Part model, mm, in its own coordinate system. Face numbers are marked on the shaded views. A direction names the side the tool comes from. Round coordinates to 2 decimals unless told otherwise and drop trailing zeros. Write each loop counter-clockwise with the first axis right and the second up, starting at its lowest first coordinate (ties: lowest second). Pieces come first, ordered by that corner, then holes.
1) Flat gauge pins, fed straight in: pin 1 (2.5 mm diameter, centred on x = -23.5, y = 23.5, fed in from -Z); pin 2 (10 mm diameter, centred on y = 4, z = 13.5, fed in from +X) (3 decimals); pin 3 (1.5 mm diameter, centred on x = -2.5, z = -27.5, fed in from +Y); pin 4 (8 mm diameter, centred on y = 6.5, z = -10.5, fed in from -X). Where does each tip first touch, or does it go through?
2) Which spindle directions (+Z, -Z, +X, -X, +Y, -Y) get a long thin tool onto all of the face, cutting with end or side? Do the marked faces 5, 6, 7 and 8. Say none if no direction does.
3) Saw through at B-B on x = 15.5. Write the cut outline in (y, z).
4) Pull direction Z, two halves, no side cores. Call the marked faces 1, 2, 3 and 4: +Z half, -Z half, draft (parallel to the pull), parting line (faces both ways), or undercut.
5) Saw through at D-D on z = 13.5. Write the cut outline in (x, y) (3 decimals), and give its area (3 significant figures).
6) Saw through at A-A on z = 6. Write the cut outline in (x, y) (3 decimals).
7) Drill centre lines: L1, parallel to Y at x = 0, z = 6 (3 decimals); L2, parallel to Y at x = -23.5, z = 2.9; L3, parallel to X at y = -23, z = 2. Where is each one in solid material? Low to high.
8) Saw through at C-C on y = 6. Write the cut outline in (x, z).
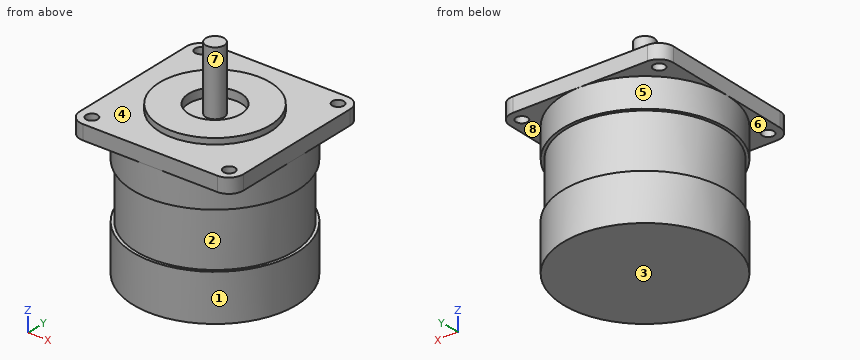
```python
from build123d import *

# Parameters (mm, degrees)
ESQUISSE1_W             = 56
ESQUISSE1_H             = 56
BOSS_EXTRU_1_DEPTH      = 5
ESQUISSE3_R             = 19
BOSS_EXTRU_2_DEPTH      = 2
ESQUISSE4_R             = 9
ENL_V_MAT_EXTRU_1_DEPTH = 3
ESQUISSE5_R             = 3.175
BOSS_EXTRU_3_DEPTH      = 22
ENL_V_MAT_EXTRU_2_REACH = 65.781
ESQUISSE6_R             = 2
CONG_1_R                = 5


with BuildPart() as part:
    # Esquisse1 → Boss.-Extru.1 (new body)
    with BuildSketch(Plane.XY):
        Rectangle(ESQUISSE1_W, ESQUISSE1_H)
    extrude(amount=BOSS_EXTRU_1_DEPTH)

    # Esquisse2 → Révolution1 (revolve)
    with BuildSketch(Plane(origin=(0, 0, 0), x_dir=(1, 0, 0), z_dir=(0, 1, 0))):
        Polygon((0, 0), (28, 0), (28, 10), (27, 10), (27, 29), (28, 29), (28, 45), (0, 45), align=None)
    revolve(axis=Axis((0, 0, 0), (0, 0, -1)))

    # Esquisse3 → Boss.-Extru.2 (add)
    with BuildSketch(Plane.XY.offset(5)):
        with Locations(Location((0, 0, 0), (0, 0, 180))):
            Circle(ESQUISSE3_R)
    extrude(amount=BOSS_EXTRU_2_DEPTH)

    # Esquisse4 → Enlèv. mat.-Extru.1 (cut)
    with BuildSketch(Plane.XY.offset(7)):
        Circle(ESQUISSE4_R)
    extrude(amount=-ENL_V_MAT_EXTRU_1_DEPTH, mode=Mode.SUBTRACT)

    # Esquisse5 → Boss.-Extru.3 (add)
    with BuildSketch(Plane.XY.offset(4)):
        Circle(ESQUISSE5_R)
    extrude(amount=BOSS_EXTRU_3_DEPTH)

    # Esquisse6 → Enlèv. mat.-Extru.2 (cut, up to next)
    with BuildSketch(Plane.XY.offset(5), mode=Mode.PRIVATE) as enl_v_mat_extru_2_sk1:
        with Locations((23.5, 23.5)):
            Circle(ESQUISSE6_R)
    enl_v_mat_extru_2_tool1 = extrude(enl_v_mat_extru_2_sk1.sketch, amount=-ENL_V_MAT_EXTRU_2_REACH, mode=Mode.PRIVATE) & part.part
    # Esquisse6 → Enlèv. mat.-Extru.2 (cut, up to next)
    with BuildSketch(Plane.XY.offset(5), mode=Mode.PRIVATE) as enl_v_mat_extru_2_sk2:
        with Locations(Location((-23.5, 23.5, 0), (0, 0, 180))):
            Circle(ESQUISSE6_R)
    enl_v_mat_extru_2_tool2 = extrude(enl_v_mat_extru_2_sk2.sketch, amount=-ENL_V_MAT_EXTRU_2_REACH, mode=Mode.PRIVATE) & part.part
    # Esquisse6 → Enlèv. mat.-Extru.2 (cut, up to next)
    with BuildSketch(Plane.XY.offset(5), mode=Mode.PRIVATE) as enl_v_mat_extru_2_sk3:
        with Locations(Location((23.5, -23.5, 0), (0, 0, 180))):
            Circle(ESQUISSE6_R)
    enl_v_mat_extru_2_tool3 = extrude(enl_v_mat_extru_2_sk3.sketch, amount=-ENL_V_MAT_EXTRU_2_REACH, mode=Mode.PRIVATE) & part.part
    # Esquisse6 → Enlèv. mat.-Extru.2 (cut, up to next)
    with BuildSketch(Plane.XY.offset(5), mode=Mode.PRIVATE) as enl_v_mat_extru_2_sk4:
        with Locations((-23.5, -23.5)):
            Circle(ESQUISSE6_R)
    enl_v_mat_extru_2_tool4 = extrude(enl_v_mat_extru_2_sk4.sketch, amount=-ENL_V_MAT_EXTRU_2_REACH, mode=Mode.PRIVATE) & part.part
    add(enl_v_mat_extru_2_tool1.solids().sort_by_distance((23.5, 23.5, 5))[0], mode=Mode.SUBTRACT)
    add(enl_v_mat_extru_2_tool2.solids().sort_by_distance((-23.5, 23.5, 5))[0], mode=Mode.SUBTRACT)
    add(enl_v_mat_extru_2_tool3.solids().sort_by_distance((23.5, -23.5, 5))[0], mode=Mode.SUBTRACT)
    add(enl_v_mat_extru_2_tool4.solids().sort_by_distance((-23.5, -23.5, 5))[0], mode=Mode.SUBTRACT)

    # Congé1
    cong_1_edges = [part.edges().sort_by_distance(p)[0] for p in [
        (-28, 28, 2.5),
        (28, 28, 2.5),
        (28, -28, 2.5),
        (-28, -28, 2.5),
    ]]
    fillet(cong_1_edges, radius=CONG_1_R)


solid = part.part
```
Completed:
1. pin 1: passes through
1. pin 2: stops at x = 3.175
1. pin 3: stops at y = 26.94
1. pin 4: stops at x = -27.89
2. face 5: -Z
2. face 6: -Z, -X, -Y
2. face 7: +Z
2. face 8: -Z, +X, +Y
3. outline: (-28, 0) - (-23.32, 0) - (-23.32, -10) - (-22.11, -10) - (-22.11, -29) - (-23.32, -29) - (-23.32, -45) - (23.32, -45) - (23.32, -29) - (22.11, -29) - (22.11, -10) - (23.32, -10) - (23.32, 0) - (28, 0) - (28, 5) - (10.99, 5) - (10.99, 7) - (-10.99, 7) - (-10.99, 5) - (-28, 5) - close
4. face 1: draft
4. face 2: undercut
4. face 3: -Z half
4. face 4: +Z half
5. outline: circle Ø6.35 at (0, 0)
5. area: 31.7 mm2
6. outline: circle Ø38 at (0, 0); circle Ø6.35 at (0, 0); hole circle Ø18 at (0, 0)
7. L1: y = -19 to -9, -3.175 to 3.175, 9 to 19
7. L2: y = -27.97 to -25.5, -21.5 to 21.5, 25.5 to 27.97
7. L3: x = -28 to -25.44, -21.56 to 21.56, 25.44 to 28
8. outline: (-28, 0) - (-27.35, 0) - (-27.35, -10) - (-26.32, -10) - (-26.32, -29) - (-27.35, -29) - (-27.35, -45) - (27.35, -45) - (27.35, -29) - (26.32, -29) - (26.32, -10) - (27.35, -10) - (27.35, 0) - (28, 0) - (28, 5) - (18.03, 5) - (18.03, 7) - (6.71, 7) - (6.71, 4) - (-6.71, 4) - (-6.71, 7) - (-18.03, 7) - (-18.03, 5) - (-28, 5) - close
